Part print with two shaded views. Sizes in mm from the minimum x, y, z corner. Round coordinates to 2 decimals unless told otherwise and drop trailing zeros. Order: outer loops, then holes, each group sorted by start corner. A loop starts at its lowest first (then second) coordinate and runs counter-clockwise, first axis right, second up. Notation, with made-up numbers: (52.5, -33.5) - (56.5, -33.5) arc R17 cw to (56.5, -6.5) - close; hole circle Ø3 at (86.5, 2). An arc over 180 degrees is marked (long way). Write item = value, one per line.
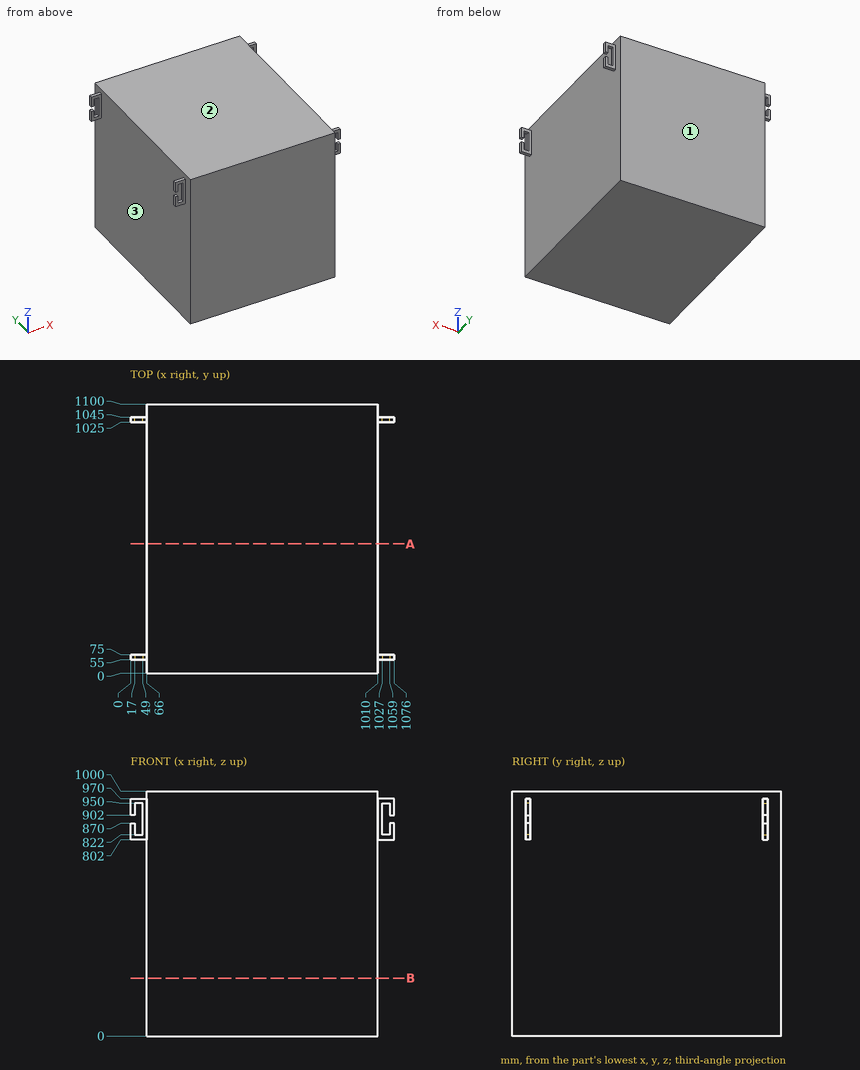
1) Flat gauge pins, fed straight in: pin 1 Ø6 at (x, y) = (447.5, 422) entering from -Z; pin 2 Ø18.5 at (x, y) = (4.5, 1030.5) entering from -Z; pin 3 Ø10 at (y, z) = (504, 376) entering from -X; pin 4 Ø10 at (x, y) = (1042, 63) entering from +Z. Where does each tip first touch, or does it go through?
Conclusion:
pin_1 = 0
pin_2 = 802
pin_3 = 66
pin_4 = 970
2) Wall check: line 1 along X through (y, z) = (888, 934). Give the ranges that are in metal, low to high.
Conclusion:
line_1 = 66 to 1010
3) Mould opens along Y. For the marked faces 1, 2 and 3 say: +Y half, -Y half, draft (parallel to the pull), parting line (faces both ways), or undercut.
Conclusion:
face_1 = +Y half
face_2 = draft
face_3 = undercut
4) Cut at A-A (y = 529). Write the cut outline in (x, z).
Conclusion:
outline = (66, 0) - (1010, 0) - (1010, 1000) - (66, 1000) - close
5) Cut at B-B (z = 236). Write the cut outline in (x, y), and give its area (3 significant figures).
Conclusion:
outline = (66, 0) - (1010, 0) - (1010, 1100) - (66, 1100) - close
area = 1,040,000 mm^2
